The model under review builds one solid part; all positions refer to its coordinate system, in mm. Give positions to 0.01 mm unless a question says otherwise; leave off trailing zeros. Order: outer loops, then holes, each group sorted by start corner. A loop starts at its lowest first (then second) coordinate and runs counter-clockwise, first axis right, second up.
```python
from build123d import *

# Parameters (mm, degrees)
BOSS_EXTRUDE1_DEPTH = 4.999999906
SKETCH3_W           = 4.999999906
SKETCH3_H           = 16.959219297
BOSS_EXTRUDE2_DEPTH = 4.999999906


with BuildPart() as part:
    # Sketch2 → Boss-Extrude1 (new body)
    with BuildSketch(Plane.XZ):
        with BuildLine():
            Line((-63.5, 63.5), (-63.5, 0))
            Line((-63.5, 0), (63.5, 0))
            Line((63.5, 0), (63.5, 63.5))
            ThreePointArc((63.5, 63.5), (0, 127), (-63.5, 63.5))
        make_face()
    extrude(amount=BOSS_EXTRUDE1_DEPTH)

    # Sketch3 → Boss-Extrude2 (add)
    with BuildSketch(Plane.XZ.offset(4.999999906)):
        with Locations((65.999999953, 8.479609649)):
            Rectangle(SKETCH3_W, SKETCH3_H)
        with Locations((65.999999953, 46.614250443)):
            Rectangle(SKETCH3_W, SKETCH3_H)
        with Locations((-65.999999953, 46.614250443)):
            Rectangle(SKETCH3_W, SKETCH3_H)
        with Locations((-65.999999953, 8.479609649)):
            Rectangle(SKETCH3_W, SKETCH3_H)
    extrude(amount=-BOSS_EXTRUDE2_DEPTH)


solid = part.part
```
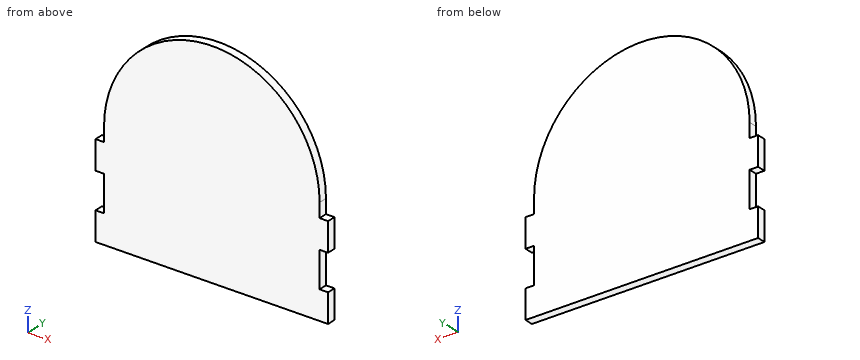
Item 1: Clearance check with flat-ended pins moving along their axes: pin 1 Ø2.5 at (y, z) = (-1.5, 24.5) entering from +X; pin 2 Ø1.5 at (x, y) = (-65.5, -3.5) entering from +Z. State where each tip first meets the part, or that it passes through.
Values found:
pin 1: stops at x = 63.5
pin 2: stops at z = 55.09
Item 2: For line 1 (X direction, y = -2.1, z = 17); line 2 (Z direction, x = 1, y = -2.3); line 3 (X direction, y = -3.9, z = 75), list the stretches that pass through material, from the lowest coordinate up.
Values found:
line 1: x = -63.5 to 63.5
line 2: z = 0 to 126.99
line 3: x = -62.45 to 62.45
Item 3: Take a section at B-B (z = 24). Give the boundary of the cut face in (x, y), and give its area (3 significant figures).
Values found:
outline: (-63.5, -5) - (63.5, -5) - (63.5, 0) - (-63.5, 0) - close
area: 635 mm2
Item 4: Take a section at A-A (y = -1.75). Give the boundary of the cut face in (x, z).
Values found:
outline: (-68.5, 0) - (68.5, 0) - (68.5, 16.96) - (63.5, 16.96) - (63.5, 38.13) - (68.5, 38.13) - (68.5, 55.09) - (63.5, 55.09) - (63.5, 63.5) arc R63.5 ccw to (-63.5, 63.5) - (-63.5, 55.09) - (-68.5, 55.09) - (-68.5, 38.13) - (-63.5, 38.13) - (-63.5, 16.96) - (-68.5, 16.96) - close
Item 5: Take a section at C-C (x = 38). Give the boundary of the cut face in (y, z), and give its area (3 significant figures).
Values found:
outline: (-5, 0) - (0, 0) - (0, 114.37) - (-5, 114.37) - close
area: 572 mm2
